CAD build for the part. Positions are in the model's coordinates, mm. Face numbers are marked on the shaded views. A direction names the side the tool comes from. Give positions to 0.01 mm unless a question says otherwise; leave off trailing zeros. Loops run counter-clockwise (first coordinate to the right, second up) from the corner with the lowest first, then second, coordinate; pieces in that order, holes last.
Item 1: Drop flat-ended pins along their axis: P1, Ø1.5, axis at x = 2, z = 4, coming from the -Y side; P2, Ø1, axis at y = 0, z = 2.5, coming from the +X side. Give the stop position or say it passes through.
Item 2: Saw through at C-C on x = -2.75. Give the cut face in (y, z).
Item 3: Saw through at D-D on y = -1.8. Give the cut face in (x, z).
Item 4: Mould opens along X. For the marked faces 3 and 4 say: released by +X, released by -X, zero draft, split by the parting line, or undercut.
Item 5: Saw through at B-B on z = 4.4. Give the cut face in (x, y), plus the area to 3 significant figures.
Item 6: Which spindle directions (+Z, -Z, +X, -X, +Y, -Y) get a long thin tool onto all of the face, cutting with end or side? Do the marked faces 1 and 2. Say none if no direction does.
Item 7: Saw through at A-A on y = -0.65. Give the cut face in (x, z), plus the area to 3 significant figures.
Item 8: Probe probe 1 along Z at (x, y) = (1, 1.6); probe 2 along Y at (x, z) = (-3, 4.05); probe 3 along X at (y, z) = (-0.65, 3.3). List the from-to ranges inside material, lowest first.
from build123d import *

# Parameters (mm, degrees)
SKETCH1_R           = 1.25
BOSS_EXTRUDE1_DEPTH = 0.5
SKETCH2_R           = 1.5
SKETCH2_R_2         = 1.25
EXTRUDE_THIN1_DEPTH = 2.5


with BuildPart() as part:
    # Sketch1 → Boss-Extrude1 (new body)
    with BuildSketch(Plane.XY):
        with BuildLine():
            Line((-3, 2.5), (3, 2.5))
            ThreePointArc((3, 2.5), (5.5, 0), (3, -2.5))
            Line((3, -2.5), (-3, -2.5))
            ThreePointArc((-3, -2.5), (-5.5, 0), (-3, 2.5))
        make_face()
        with Locations((-3, 0)):
            Circle(SKETCH1_R, mode=Mode.SUBTRACT)
        with Locations((3, 0)):
            Circle(SKETCH1_R, mode=Mode.SUBTRACT)
    boss_extrude1 = extrude(amount=BOSS_EXTRUDE1_DEPTH)

    # Sketch2 → Extrude-Thin1 (add)
    # profile 1 of 2: a face of its own
    with BuildSketch(Plane.XY.offset(0.5)):
        with Locations((-3, 0)):
            Circle(SKETCH2_R)
        with Locations((-3, 0)):
            Circle(SKETCH2_R_2, mode=Mode.SUBTRACT)
    # profile 2 of 2: a face of its own
    with BuildSketch(Plane.XY.offset(0.5)):
        with Locations((3, 0)):
            Circle(SKETCH2_R)
        with Locations((3, 0)):
            Circle(SKETCH2_R_2, mode=Mode.SUBTRACT)
    extrude_thin1 = extrude(amount=EXTRUDE_THIN1_DEPTH)

    # Mirror1: Boss-Extrude1, Extrude-Thin1 across plane
    add(boss_extrude1.mirror(Plane.XY.offset(3)))
    add(extrude_thin1.mirror(Plane.XY.offset(3)))


solid = part.part
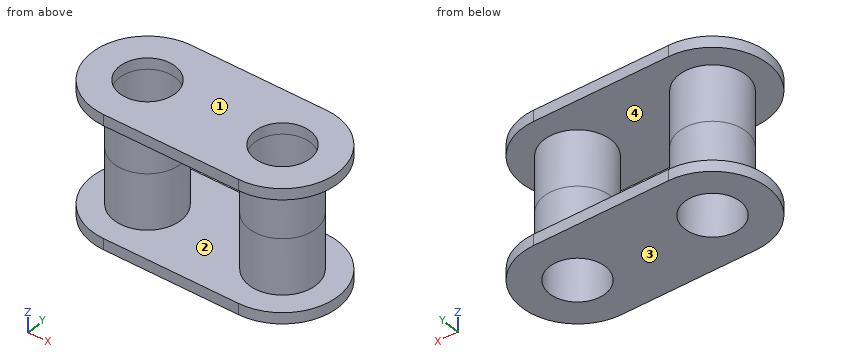
Results below:
1. P1: stops at y = -1.48
1. P2: stops at x = 4.5
2. outline: (-2.5, 0) - (-1.22, 0) - (-1.22, 6) - (-2.5, 6) - (-2.5, 5.5) - (-1.48, 5.5) - (-1.48, 0.5) - (-2.5, 0.5) - close; (1.22, 0) - (2.5, 0) - (2.5, 0.5) - (1.48, 0.5) - (1.48, 5.5) - (2.5, 5.5) - (2.5, 6) - (1.22, 6) - close
3. outline: (-4.73, 0) - (4.73, 0) - (4.73, 0.5) - (-4.73, 0.5) - close; (-4.73, 5.5) - (4.73, 5.5) - (4.73, 6) - (-4.73, 6) - close
4. face 3: zero draft
4. face 4: undercut
5. outline: circle Ø3 at (-3, 0); circle Ø3 at (3, 0); hole circle Ø2.5 at (-3, 0); hole circle Ø2.5 at (3, 0)
5. area: 4.32 mm2
6. face 1: +Z, +X, -X, +Y, -Y
6. face 2: none
7. outline: (-5.41, 0) - (-4.07, 0) - (-4.07, 6) - (-5.41, 6) - (-5.41, 5.5) - (-4.35, 5.5) - (-4.35, 0.5) - (-5.41, 0.5) - close; (-1.93, 0) - (1.93, 0) - (1.93, 6) - (-1.93, 6) - close; (4.07, 0) - (5.41, 0) - (5.41, 0.5) - (4.35, 0.5) - (4.35, 5.5) - (5.41, 5.5) - (5.41, 6) - (4.07, 6) - close; hole (-1.65, 0.5) - (1.65, 0.5) - (1.65, 5.5) - (-1.65, 5.5) - close
7. area: 12.2 mm2
8. probe 1: z = 0 to 0.5, 5.5 to 6
8. probe 2: y = -1.5 to -1.25, 1.25 to 1.5
8. probe 3: x = -4.35 to -4.07, -1.93 to -1.65, 1.65 to 1.93, 4.07 to 4.35
